Geometry: final body of the model. Coordinates: model frame, mm. Give positions to 0.01 mm unless a question says otherwise; leave off trailing zeros. Order: outer loops, then holes, each group sorted by start corner. A loop starts at its lowest first (then second) coordinate and runs counter-clockwise, first axis right, second up. Notation, with made-up numbers: (56, 67.25) -> (92, 67.25) arc R9 ccw to (92, 74.25) -> close; hole circle Ø9 at (-11, 52). An arc over 180 degrees is marked (long way). One line per question, with ' | ' between items. Start each with the question number.
(1) Section B-B (y = 10). Return loops of the section in (x, z), then the cut area to 3 significant figures.
(2) Section C-C (x = 75). Return loops of the section in (y, z).
(3) Section D-D (x = 40). State how many separate pieces and enclosed holes the cut face has, then the cut area to 3 significant figures.
(4) Ray query, L1, parallel to X at y = 54, z = 0.9; L2, parallel to Y at x = 41, z = 0.5; L3, parallel to Y at x = 42, z = 1.6. Return the intervals inside material, ascending.
(5) First-contact query: pin 1 Ø3.5 at (x, y) = (41, 54) entering from +Z; pin 2 Ø10 at (x, y) = (30.5, 13) entering from -Z. Flat tips, straight axial feed; report the tip coordinate or a pass-through.
(6) Mould query, pull axis Y, two halves, no side actions, for faces 1 (the face through (74, 64, 1)), 2 (the face through (110.642, 56.727, 0.567)), 3 (the face through (49, 0, 1)), 4 (the face through (0, 32, 1)). Classes: +Y half, -Y half, draft (parallel to the pull), parting line (faces both ways), or undercut.
(7) Section A-A (z = 1.75). Return loops of the section in (x, y).
```python
from build123d import *

# Parameters (mm, degrees)
SKETCH1_R                                            = 2.75
BOSS_EXTRUDE1_DEPTH                                  = 4
FILLET1_R                                            = 1
CSK_FOR_M5_HEX_SOCKET_COUNTERSUNK_CAP_SC_D           = 5.5
CSK_FOR_M5_HEX_SOCKET_COUNTERSUNK_CAP_SC_DEPTH       = 12.4
CSK_FOR_M5_HEX_SOCKET_COUNTERSUNK_CAP_SC_CSINK_D     = 11.2
CSK_FOR_M5_HEX_SOCKET_COUNTERSUNK_CAP_SC_CSINK_ANGLE = 90
CSK_FOR_M5_HEX_SOCKET_COUNTERSUNK_CAP_SC_TIP         = 1.652366702


with BuildPart() as part:
    # Sketch1 → Boss-Extrude1 (new body)
    with BuildSketch(Plane.XY):
        Polygon((0, 0), (0, 64), (151, 64), (151, -30), (121, -30), (95.827011065, 0), align=None)
        with Locations((41, 54)):
            Circle(SKETCH1_R, mode=Mode.SUBTRACT)
        with Locations((111, 54)):
            Circle(SKETCH1_R, mode=Mode.SUBTRACT)
        with Locations((40, 10)):
            Circle(SKETCH1_R, mode=Mode.SUBTRACT)
    extrude(amount=BOSS_EXTRUDE1_DEPTH)

    # Fillet1
    fillet1_edges = [part.edges().sort_by_distance(p)[0] for p in [
        (136, -30, 4),
        (151, 17, 4),
        (75.5, 64, 4),
        (0, 32, 4),
        (47.913505532, 0, 4),
        (108.413505532, -15, 4),
    ]]
    fillet(fillet1_edges, radius=FILLET1_R)

    # CSK for M5 Hex Socket Countersunk Cap Screw1
    with Locations(Plane.XY.offset(4)):
        with Locations((41, 54), (111, 54), (40, 10)):
            CounterSinkHole(CSK_FOR_M5_HEX_SOCKET_COUNTERSUNK_CAP_SC_D / 2, CSK_FOR_M5_HEX_SOCKET_COUNTERSUNK_CAP_SC_CSINK_D / 2, depth=CSK_FOR_M5_HEX_SOCKET_COUNTERSUNK_CAP_SC_DEPTH, counter_sink_angle=CSK_FOR_M5_HEX_SOCKET_COUNTERSUNK_CAP_SC_CSINK_ANGLE)
            with Locations((0, 0, -(CSK_FOR_M5_HEX_SOCKET_COUNTERSUNK_CAP_SC_DEPTH + CSK_FOR_M5_HEX_SOCKET_COUNTERSUNK_CAP_SC_TIP / 2))):  # 118° drill point
                Cone(0, CSK_FOR_M5_HEX_SOCKET_COUNTERSUNK_CAP_SC_D / 2, CSK_FOR_M5_HEX_SOCKET_COUNTERSUNK_CAP_SC_TIP, mode=Mode.SUBTRACT)


solid = part.part
```
Response:
1) outline: (0, 0) -> (37.25, 0) -> (37.25, 1.15) -> (34.4, 4) -> (1, 4) arc R1 ccw to (0, 3) -> close; (42.75, 0) -> (151, 0) -> (151, 3) arc R1 ccw to (150, 4) -> (45.6, 4) -> (42.75, 1.15) -> close | area: 573 mm^2
2) outline: (0, 0) -> (64, 0) -> (64, 3) arc R1 ccw to (63, 4) -> (1, 4) arc R1 ccw to (0, 3) -> close
3) separate pieces: 3 | enclosed holes: 0 | area: 196 mm^2
4) L1: x = 0 to 38.25, 43.75 to 108.25, 113.75 to 151 | L2: y = 0 to 7.44, 12.56 to 51.25, 56.75 to 64 | L3: y = 0 to 7.5, 12.5 to 50.96, 57.04 to 64
5) pin 1: passes through | pin 2: stops at z = 0
6) face 1: +Y half | face 2: undercut | face 3: -Y half | face 4: draft
7) outline: (0, 0) -> (95.83, 0) -> (121, -30) -> (151, -30) -> (151, 64) -> (0, 64) -> close; hole circle Ø6.7 at (40, 10); hole circle Ø6.7 at (41, 54); hole circle Ø6.7 at (111, 54)
